Design review of the part built by this model. Coordinates are the model's own, in mm. A direction names the side the tool comes from. Coordinates: 2 decimals unless noted, no trailing zeros. Order: outer loops, then holes, each group sorted by start corner. A loop starts at its lowest first (then second) coordinate and runs counter-clockwise, first axis right, second up. Notation, with made-up numbers: M 89,-7.75 L 98,-7.75 A18 cw 98,13.25 Z; hole C 78,43.25 d11. An arc over 180 degrees is marked long. Answer as a JSON object with one key per item and string values.
Solid Edge part; units mm, degrees
sketch "Sketch1" plane through (0, 0, 0) normal (0, 0, 1) x (1, 0, 0)
  circle A0 centre (38.0952, 31.3095) radius 25
extrude "Protrusion1" add sketch "Sketch1" along normal blind 50
sketch "Sketch2" plane through (38.0952, 31.3095, 50) normal (0, 0, 1) x (1, 0, 0)
  line L0 (-16, 16) -> (16, 16)
  line L1 (16, 16) -> (16, -16)
  line L2 (16, -16) -> (-16, -16)
  line L3 (-16, -16) -> (-16, 16)
  dimension "D1" = 16
  dimension "D2" = 16
extrude "ExtrudedProtrusion_2" add sketch "Sketch2" along normal blind 50
hole "Hole_1" at (22.0952, 31.3095, 85) direction (1, 0, 0) diameter 10 end through all
hole "Hole1" at (22.0952, 31.3095, 65) direction (1, 0, 0) diameter 10 end through all
hole "Hole_2" at (38.0952, 31.3095, 0) direction (0, 0, 1) diameter 17.294 depth 25 tip angle 118 thread major 20 thread length 20
chamfer "Chamfer_1" distance 2 angle 45 1 edges at (38.0952, 22.6625, 0)
chamfer "Chamfer_2" distance 1 angle 45 1 edges at (13.0952, 31.3095, 0)
chamfer "Chamfer_3" distance 1 angle 45 1 edges at (13.0952, 31.3095, 50)
chamfer "Chamfer_4" distance 1 angle 45 2 edges at (22.0952, 31.3095, 80) (54.0952, 26.3095, 85)
chamfer "Chamfer_5" distance 1 angle 45 2 edges at (22.0952, 31.3095, 60) (54.0952, 26.3095, 65)
1) Insertion check: pin 1 Ø4 at (y, z) = (35.5, 60.5) entering from -X; pin 2 Ø10 at (y, z) = (37, 38.5) entering from +X; pin 3 Ø9.5 at (y, z) = (38, 79) entering from +X. Each pin has a flat end and moves straight along its axis. Give the tip position at first contact, or say it passes through.
Taken from the geometry:
{"pin 1": "stops at x = 22.1", "pin 2": "stops at x = 63.09", "pin 3": "stops at x = 54.1"}
2) To check wall thickness, follow L1, parallel to Y at x = 45, z = 65; L2, parallel to Z at x = 32, y = 30.5; L3, parallel to Z at x = 20.5, y = 40. State the ranges of each line that lie inside material, in increasing order.
Taken from the geometry:
{"L1": "y = 15.31 to 26.31, 36.31 to 47.31", "L2": "z = 26.5 to 60.07, 69.93 to 80.07, 89.93 to 100", "L3": "z = 0 to 50"}
3) Add section C-C (z = 7.5). State the section outline as (x, y) points.
Taken from the geometry:
{"outline": "C 38.1,31.31 d50; hole C 38.1,31.31 d17.29"}
4) Tool access review of faces 4 (the flat face through (38, 47.31, 75)), 5 (the flat face through (38, 15.31, 75)), 6 (the cylindrical face through (41.4, 39.3, 13.7)), 7 (the flat face through (22.095, 31, 75)), 8 (the flat face through (54.095, 32, 75)): name each direction out of +Z, -Z, +X, -X, +Y, -Y from which nothing blocks a thin tool from reaching the whole face with its end or side.
Taken from the geometry:
{"face 4": "+Z, +X, -X, +Y", "face 5": "+Z, +X, -X, -Y", "face 6": "-Z", "face 7": "+Z, -X, +Y, -Y", "face 8": "+Z, +X, +Y, -Y"}
5) Add section B-B (x = 45). Count the separate pieces of the cut face and the enclosed holes in it, and give its area (3 significant figures).
Taken from the geometry:
{"separate pieces": "1", "enclosed holes": "2", "area": "3,570 mm2"}
6) Mouldability with a two-part tool opening along Y and no side actions: class faces 1 (the cylindrical face through (61.94, 23.8, 24.66)), 2 (the flat face through (38, 32, 100)), 3 (the cylindrical face through (37.885, 35.526, 87.688)) as released by +Y, released by -Y, zero draft, split by the parting line, or undercut.
Taken from the geometry:
{"face 1": "split by the parting line", "face 2": "zero draft", "face 3": "undercut"}
7) Add section A-A (z = 65). State the section outline as (x, y) points.
Taken from the geometry:
{"outline": "M 22.1,15.31 L 54.1,15.31 L 54.1,25.31 L 53.1,26.31 L 23.1,26.31 L 22.1,25.31 Z; M 22.1,37.31 L 23.1,36.31 L 53.1,36.31 L 54.1,37.31 L 54.1,47.31 L 22.1,47.31 Z"}
